```python
from build123d import *

# Parameters (mm, degrees)
BOSS_EXTRUDE1_DEPTH = 152.4
SKETCH2_R           = 1.190625
SKETCH2_W           = 19.84375
SKETCH2_H           = 39.6875
CUT_EXTRUDE1_DEPTH  = 6.35
CUT_EXTRUDE2_DEPTH  = 2.38125
CUT_EXTRUDE3_DEPTH  = 2.38125
BOSS_EXTRUDE2_DEPTH = 2.38125
BOSS_EXTRUDE3_DEPTH = 2.38125
FILLET1_R           = 2.54
SKETCH7_W           = 51.674409632
SKETCH7_H           = 14.688438898
CUT_EXTRUDE4_DEPTH  = 172.100000261
FILLET2_R           = 8.89
SKETCH8_R           = 3.96875
CUT_EXTRUDE5_DEPTH  = 170.479485102
CUT_EXTRUDE6_DEPTH  = 169.363218031


with BuildPart() as part:
    # Sketch1 → Boss-Extrude1 (new body)
    with BuildSketch(Plane(origin=(0, 0, 0), x_dir=(1, 0, 0), z_dir=(0, 1, 0))):
        Polygon((-38.941593287, 17.493761907), (21.383406713, 17.493761907), (21.383406713, -25.368738093), (16.620906713, -25.368738093), (16.620906713, 12.731261907), (-34.179093287, 12.731261907), (-34.179093287, -25.368738093), (-38.941593287, -25.368738093), align=None)
    extrude(amount=BOSS_EXTRUDE1_DEPTH)

    # Sketch2 → Cut-Extrude1 (cut)
    with BuildSketch(Plane(origin=(21.383406713, 0, 0), x_dir=(0, 0, -1), z_dir=(1, 0, 0))):
        with Locations((-11.478113093, 14.2875)):
            Circle(SKETCH2_R)
        with Locations((-1.159363093, 14.2875)):
            Circle(SKETCH2_R)
        with Locations((-1.159363093, 61.9125)):
            Circle(SKETCH2_R)
        with Locations((-11.478113093, 61.9125)):
            Circle(SKETCH2_R)
        with Locations((-6.318738093, 38.1)):
            Rectangle(SKETCH2_W, SKETCH2_H)
    extrude(amount=-CUT_EXTRUDE1_DEPTH, mode=Mode.SUBTRACT)

    # Sketch3 → Cut-Extrude2 (cut)
    with BuildSketch(Plane(origin=(21.383406713, 0, 0), x_dir=(0, 0, -1), z_dir=(1, 0, 0))):
        Polygon((-20.587285527, 5.690264064), (-9.47039523, 5.690264064), (-12.431175058, 0), (-17.905824551, 0), align=None)
        Polygon((-0.206301127, 0), (5.268348366, 0), (7.949809342, 5.690264064), (-3.167080955, 5.690264064), align=None)
    extrude(amount=-CUT_EXTRUDE2_DEPTH, mode=Mode.SUBTRACT)

    # Sketch4 → Cut-Extrude3 (cut)
    with BuildSketch(Plane(origin=(-34.179093287, 0, 0), x_dir=(0, 0, -1), z_dir=(1, 0, 0))):
        Polygon((-9.47039523, 5.690264064), (-20.587285527, 5.690264064), (-17.905824551, 0), (-12.431175058, 0), align=None)
        Polygon((5.268348366, 0), (7.949809342, 5.690264064), (-3.167080955, 5.690264064), (-0.206301127, 0), align=None)
    extrude(amount=-CUT_EXTRUDE3_DEPTH, mode=Mode.SUBTRACT)

    # Sketch5 → Boss-Extrude2 (add)
    with BuildSketch(Plane(origin=(21.383406713, 0, 0), x_dir=(0, 0, -1), z_dir=(1, 0, 0))):
        Polygon((-0.206301127, 152.4), (5.268348366, 152.4), (7.949809342, 158.090264064), (-3.167080955, 158.090264064), align=None)
        Polygon((-17.905824551, 152.4), (-12.431175058, 152.4), (-9.47039523, 158.090264064), (-20.587285527, 158.090264064), align=None)
    extrude(amount=-BOSS_EXTRUDE2_DEPTH)

    # Sketch6 → Boss-Extrude3 (add)
    with BuildSketch(Plane(origin=(-34.179093287, 0, 0), x_dir=(0, 0, -1), z_dir=(1, 0, 0))):
        Polygon((-17.905824551, 152.4), (-12.431175058, 152.4), (-9.47039523, 158.090264064), (-20.587285527, 158.090264064), align=None)
        Polygon((5.268348366, 152.4), (7.949809342, 158.090264064), (-3.167080955, 158.090264064), (-0.206301127, 152.4), align=None)
    extrude(amount=-BOSS_EXTRUDE3_DEPTH)

    # Fillet1
    fillet1_edges = [part.edges().sort_by_distance(p)[0] for p in [
        (-36.560343287, 0, 25.368738093),
        (-38.941593287, 76.2, -17.493761907),
        (21.383406713, 76.2, -17.493761907),
        (19.002156713, 152.4, 25.368738093),
        (-36.560343287, 152.4, 25.368738093),
        (19.002156713, 0, 25.368738093),
    ]]
    fillet(fillet1_edges, radius=FILLET1_R)

    # Sketch7 → Cut-Extrude4 (cut, through all)
    with BuildSketch(Plane(origin=(21.383406713, 0, 0), x_dir=(0, 0, -1), z_dir=(1, 0, 0))):
        with Locations((-4.704390425, 2.848923491)):
            Rectangle(SKETCH7_W, SKETCH7_H)
    extrude(amount=-CUT_EXTRUDE4_DEPTH, mode=Mode.SUBTRACT)

    # Fillet2
    fillet2_edges = [part.edges().sort_by_distance(p)[0] for p in [
        (-36.560343287, 10.19314294, 25.368738093),
        (19.002156713, 10.19314294, 25.368738093),
    ]]
    fillet(fillet2_edges, radius=FILLET2_R)

    # Sketch8 → Cut-Extrude5 (cut, through all)
    with BuildSketch(Plane(origin=(-34.179093287, 0, 0), x_dir=(0, 0, -1), z_dir=(1, 0, 0))):
        with Locations((-6.318738093, 26.9875)):
            Circle(SKETCH8_R)
    extrude(amount=-CUT_EXTRUDE5_DEPTH, mode=Mode.SUBTRACT)

    # Sketch9 → Cut-Extrude6 (cut, through all)
    with BuildSketch(Plane(origin=(0, 0, -17.493761907), x_dir=(-1, 0, 0), z_dir=(0, 0, -1))):
        Polygon((8.201765803, 131.642746086), (12.926215978, 134.370408666), (12.926215978, 139.825733827), (8.201765803, 142.553396407), (3.477315628, 139.825733827), (3.477315628, 134.370408666), align=None)
        Polygon((-10.086234197, 131.642746086), (-5.361784022, 134.370408666), (-5.361784022, 139.825733827), (-10.086234197, 142.553396407), (-14.810684372, 139.825733827), (-14.810684372, 134.370408666), align=None)
        Polygon((26.489765803, 131.642746086), (31.214215978, 134.370408666), (31.214215978, 139.825733827), (26.489765803, 142.553396407), (21.765315628, 139.825733827), (21.765315628, 134.370408666), align=None)
        Polygon((8.201765803, 106.242746086), (12.926215978, 108.970408666), (12.926215978, 114.425733827), (8.201765803, 117.153396407), (3.477315628, 114.425733827), (3.477315628, 108.970408666), align=None)
        Polygon((26.489765803, 106.242746086), (31.214215978, 108.970408666), (31.214215978, 114.425733827), (26.489765803, 117.153396407), (21.765315628, 114.425733827), (21.765315628, 108.970408666), align=None)
        Polygon((8.201765803, 80.842746086), (12.926215978, 83.570408666), (12.926215978, 89.025733827), (8.201765803, 91.753396407), (3.477315628, 89.025733827), (3.477315628, 83.570408666), align=None)
        Polygon((26.489765803, 80.842746086), (31.214215978, 83.570408666), (31.214215978, 89.025733827), (26.489765803, 91.753396407), (21.765315628, 89.025733827), (21.765315628, 83.570408666), align=None)
        Polygon((8.201765803, 55.442746086), (12.926215978, 58.170408666), (12.926215978, 63.625733827), (8.201765803, 66.353396407), (3.477315628, 63.625733827), (3.477315628, 58.170408666), align=None)
        Polygon((26.489765803, 55.442746086), (31.214215978, 58.170408666), (31.214215978, 63.625733827), (26.489765803, 66.353396407), (21.765315628, 63.625733827), (21.765315628, 58.170408666), align=None)
        Polygon((8.201765803, 30.042746086), (12.926215978, 32.770408666), (12.926215978, 38.225733827), (8.201765803, 40.953396407), (3.477315628, 38.225733827), (3.477315628, 32.770408666), align=None)
        Polygon((26.489765803, 30.042746086), (31.214215978, 32.770408666), (31.214215978, 38.225733827), (26.489765803, 40.953396407), (21.765315628, 38.225733827), (21.765315628, 32.770408666), align=None)
        Polygon((-10.086234197, 106.242746086), (-5.361784022, 108.970408666), (-5.361784022, 114.425733827), (-10.086234197, 117.153396407), (-14.810684372, 114.425733827), (-14.810684372, 108.970408666), align=None)
        Polygon((-10.086234197, 80.842746086), (-5.361784022, 83.570408666), (-5.361784022, 89.025733827), (-10.086234197, 91.753396407), (-14.810684372, 89.025733827), (-14.810684372, 83.570408666), align=None)
        Polygon((-10.086234197, 55.442746086), (-5.361784022, 58.170408666), (-5.361784022, 63.625733827), (-10.086234197, 66.353396407), (-14.810684372, 63.625733827), (-14.810684372, 58.170408666), align=None)
        Polygon((-10.086234197, 30.042746086), (-5.361784022, 32.770408666), (-5.361784022, 38.225733827), (-10.086234197, 40.953396407), (-14.810684372, 38.225733827), (-14.810684372, 32.770408666), align=None)
    extrude(amount=-CUT_EXTRUDE6_DEPTH, mode=Mode.SUBTRACT)


solid = part.part
```
Could you check a few things on this model? Use its own coordinates, in mm. A direction names the side the tool comes from. Round coordinates to 2 decimals unless told otherwise and drop trailing zeros. Write each loop counter-clockwise with the first axis right and the second up, starting at its lowest first coordinate (ties: lowest second). Pieces come first, ordered by that corner, then holes.
(1) Suppose I cut it at A-A on y = 53. Write out the boundary of the cut face in (x, z), and give its area (3 significant figures).
Findings below:
outline: (-38.94, -14.95) arc R2.54 ccw to (-36.4, -17.49) - (18.84, -17.49) arc R2.54 ccw to (21.38, -14.95) - (21.38, -3.6) - (16.62, -3.6) - (16.62, -12.73) - (-34.18, -12.73) - (-34.18, 25.37) - (-38.94, 25.37) - close; (16.62, 16.24) - (21.38, 16.24) - (21.38, 25.37) - (16.62, 25.37) - close
area: 553 mm2
(2) Suppose I cut it at C-C on z = -1.5. Write out the boundary of the cut face in (x, y).
Findings below:
outline: (-38.94, 10.19) - (-34.18, 10.19) - (-34.18, 158.09) - (-36.56, 158.09) - (-36.56, 152.4) - (-38.94, 152.4) - close; (16.62, 10.19) - (21.38, 10.19) - (21.38, 18.26) - (16.62, 18.26) - close; (16.62, 57.94) - (21.38, 57.94) - (21.38, 158.09) - (19, 158.09) - (19, 152.4) - (16.62, 152.4) - close
(3) Which directions (+Z, -Z, +X, -X, +Y, -Y) give clear straight access to the entire face, cutting with the end or side of a thin tool? Please do faces 1 (the face through (-35.353, 155.285, 19.265)), 2 (the face through (-3.477, 112, -15)), 3 (the face through (19.002, 156, -2)).
Findings below:
face 1: +Z, +X, -X
face 2: +Z, -Z
face 3: +Z, -Z, +Y
(4) Suppose I cut it at B-B on z = -11. Write out the boundary of the cut face in (x, y).
Findings below:
outline: (-38.94, 10.19) - (-34.18, 10.19) - (-34.18, 152.4) - (-38.94, 152.4) - close; (16.62, 10.19) - (21.38, 10.19) - (21.38, 152.4) - (16.62, 152.4) - close
(5) For pin 1 (3 mm diameter, centred on x = 10, y = 72, fed in from +Z); pin 2 (8 mm diameter, centred on x = -12, z = -11, fed in from +Y); pin 3 (1.5 mm diameter, centred on y = 32.5, z = 1.5, fed in from +X), each with a flat end and sliding along its axis, tell me the tip position at first contact or that it passes through.
Findings below:
pin 1: stops at z = -12.73
pin 2: stops at y = 152.4
pin 3: stops at x = -34.18
(6) If I drill on probe 1 along X at (y, z) = (134.5, -13); probe 2 along X at (y, z) = (123.5, -4); probe 3 along X at (y, z) = (25, 16), over which ranges is the centre line in solid material (lowest first)?
Findings below:
probe 1: x = -38.94 to -31.21, -21.77 to -12.93, -3.48 to 5.36, 14.81 to 21.38
probe 2: x = -38.94 to -34.18, 16.62 to 21.38
probe 3: x = -38.94 to -34.18
(7) Thinking about a two-plate mould opening in X: for faces 4 (the face through (12.482, 133.026, -15.146)), 5 (the face through (-38.942, 80, 5)), 6 (the face through (-37, 84, 25.369)), 7 (the face through (-28.82, 31.39, -15.15)), which applies, +X half, -X half, draft (parallel to the pull), parting line (faces both ways), or undercut?
Findings below:
face 4: undercut
face 5: -X half
face 6: draft
face 7: undercut
(8) Suppose I cut it at D-D on y = 97. Write out the boundary of the cut face in (x, z).
Findings below:
outline: (-38.94, -14.95) arc R2.54 ccw to (-36.4, -17.49) - (18.84, -17.49) arc R2.54 ccw to (21.38, -14.95) - (21.38, 25.37) - (16.62, 25.37) - (16.62, -12.73) - (-34.18, -12.73) - (-34.18, 25.37) - (-38.94, 25.37) - close
